```python
from build123d import *

# Parameters (mm, degrees)
CROQUIS2_R              = 1.5
CROQUIS2_R_2            = 10
SALIENTE_EXTRUIR2_DEPTH = 3
CROQUIS4_W              = 8
CROQUIS4_H              = 6
CORTAR_EXTRUIR1_DEPTH   = 32.960913629


with BuildPart() as part:
    # Croquis2 → Saliente-Extruir2 (new body)
    with BuildSketch(Plane.XY):
        with BuildLine():
            ThreePointArc((-4.305099018, -20.042857143), (0, -22.5), (4.305099018, -20.042857143))
            ThreePointArc((4.305099018, -20.042857143), (14.495689014, -14.495689014), (20.042857143, -4.305099018))
            ThreePointArc((20.042857143, -4.305099018), (22.5, 0), (20.042857143, 4.305099018))
            ThreePointArc((20.042857143, 4.305099018), (14.495689014, 14.495689014), (4.305099018, 20.042857143))
            ThreePointArc((4.305099018, 20.042857143), (0, 22.5), (-4.305099018, 20.042857143))
            ThreePointArc((-4.305099018, 20.042857143), (-14.495689014, 14.495689014), (-20.042857143, 4.305099018))
            ThreePointArc((-20.042857143, 4.305099018), (-22.5, 0), (-20.042857143, -4.305099018))
            ThreePointArc((-20.042857143, -4.305099018), (-14.495689014, -14.495689014), (-4.305099018, -20.042857143))
        make_face()
        with BuildLine():
            ThreePointArc((-15.121652909, -5.228347091), (-8.661165235, -8.661165235), (-5.228347091, -15.121652909))
            ThreePointArc((-5.228347091, -15.121652909), (-11.313708499, -11.313708499), (-15.121652909, -5.228347091))
        make_face(mode=Mode.SUBTRACT)
        with Locations((0, -17.5)):
            Circle(CROQUIS2_R, mode=Mode.SUBTRACT)
        with BuildLine():
            ThreePointArc((15.121652909, -5.228347091), (11.313708499, -11.313708499), (5.228347091, -15.121652909))
            ThreePointArc((5.228347091, -15.121652909), (8.661165235, -8.661165235), (15.121652909, -5.228347091))
        make_face(mode=Mode.SUBTRACT)
        with Locations((-17.5, 0)):
            Circle(CROQUIS2_R, mode=Mode.SUBTRACT)
        with BuildLine():
            ThreePointArc((-15.121652909, 5.228347091), (-11.313708499, 11.313708499), (-5.228347091, 15.121652909))
            ThreePointArc((-5.228347091, 15.121652909), (-8.661165235, 8.661165235), (-15.121652909, 5.228347091))
        make_face(mode=Mode.SUBTRACT)
        Circle(CROQUIS2_R_2, mode=Mode.SUBTRACT)
        with Locations((17.5, 0)):
            Circle(CROQUIS2_R, mode=Mode.SUBTRACT)
        with Locations((0, 17.5)):
            Circle(CROQUIS2_R, mode=Mode.SUBTRACT)
        with BuildLine():
            ThreePointArc((5.228347091, 15.121652909), (11.313708499, 11.313708499), (15.121652909, 5.228347091))
            ThreePointArc((15.121652909, 5.228347091), (8.661165235, 8.661165235), (5.228347091, 15.121652909))
        make_face(mode=Mode.SUBTRACT)
    extrude(amount=SALIENTE_EXTRUIR2_DEPTH)

    # Croquis4 → Cortar-Extruir1 (cut, through all)
    with BuildSketch(Plane(origin=(0, 0, 0), x_dir=(-1, 0, 0), z_dir=(0, 0, -1))):
        with Locations((-10, 0)):
            Rectangle(CROQUIS4_W, CROQUIS4_H)
    extrude(amount=-CORTAR_EXTRUIR1_DEPTH, mode=Mode.SUBTRACT)


solid = part.part
```
Can you work these out from the model? Positions are in its coordinate system, mm. A direction names the side the tool comes from. Round coordinates to 2 decimals unless told otherwise and drop trailing zeros. Loops run counter-clockwise (first coordinate to the right, second up) from the corner with the lowest first, then second, coordinate; pieces in that order, holes last. Notation, with made-up numbers: M 65,-21 L 102,-21 A32 cw 102,6 Z; hole C 56.5,55 d6. An arc over 180 degrees is marked long. Answer as a JSON object with one key per item and string values. Group by question number.
Q1. Imagine slicing it at D-D, the plane x = -11. Please give me the cut outline in (y, z), then the cut area to 3 significant figures.
Q2. Imagine slicing it at C-C, the plane y = -17.5. Please give me the cut outline in (x, z), then the cut area to 3 significant figures.
Q3. Will these pins go through, and if not, where does the flat tip stop? pin 1 (12 mm diameter, centred on x = 0.5, y = 6.5, fed in from -Z); pin 2 (0.9 mm diameter, centred on x = 10.5, z = 2, fed in from -Y); pin 3 (1.5 mm diameter, centred on x = 11.5, z = 1.5, fed in from +Y); pin 4 (1.5 mm diameter, centred on x = -5.5, z = 1.5, fed in from -Y).
Q4. Please list where these lines run through material, in increasing order: L1, parallel to Y at x = -6.5, z = 0.3; L2, parallel to X at y = 8, z = 1.95; L3, parallel to Y at x = -1, z = 1.95.
Q5. We'd pull the mould along X, two halves only. Please class faces 1 (the cylindrical face through (0, 19, 1)), 2 (the cylindrical face through (22.5, -0.1, 1.5)), 3 (the cylindrical face through (-14.38, 14.61, 1.48)): +X half, -X half, draft (parallel to the pull), parting line (faces both ways), or undercut.
Q6. On a 3-axis mill with a long thin cutter (end or side, diameter ignored), from which of +Z, -Z, +X, -X, +Y, -Y can I reach the whole of each face in a straight line? I mean faces 4 (the cylindrical face through (14.38, -14.61, 1.48)), 5 (the flat face through (14, 0, 1)). Say none if no direction works.
Q7. Imagine slicing it at A-A, the plane z = 0.75. Count the separate pieces of the cut face and the enclosed holes in it, then the cut area to 3 significant figures.
Q8. Imagine slicing it at B-B, the plane x = 0. Please give me the cut outline in (y, z).
Findings:
{
 "1": {"outline": "M -17.3,0 L -11.62,0 L -11.62,3 L -17.3,3 Z; M -6.82,0 L 6.82,0 L 6.82,3 L -6.82,3 Z; M 11.62,0 L 17.3,0 L 17.3,3 L 11.62,3 Z", "area": "75.0 mm2"},
 "2": {"outline": "M -10.68,0 L -1.5,0 L -1.5,3 L -10.68,3 Z; M 1.5,0 L 10.68,0 L 10.68,3 L 1.5,3 Z", "area": "55.1 mm2"},
 "3": {"pin 1": "stops at z = 0", "pin 2": "stops at y = -17.87", "pin 3": "stops at y = 17.46", "pin 4": "stops at y = -19.94"},
 "4": {"L1": "y = -19.44 to -14.62, -11.56 to -7.6, 7.6 to 11.56, 14.62 to 19.44", "L2": "x = -18.87 to -13.86, -9.38 to -6, 6 to 9.38, 13.86 to 18.87", "L3": "y = -22.4 to -18.62, -16.38 to -9.95, 9.95 to 16.38, 18.62 to 22.4"},
 "5": {"face 1": "undercut", "face 2": "+X half", "face 3": "-X half"},
 "6": {"face 4": "+Z, -Z, +X, -Y", "face 5": "+Z, -Z"},
 "7": {"separate pieces": "1", "enclosed holes": "9", "area": "860 mm2"},
 "8": {"outline": "M -22.5,0 L -19,0 L -19,3 L -22.5,3 Z; M -16,0 L -10,0 L -10,3 L -16,3 Z; M 10,0 L 16,0 L 16,3 L 10,3 Z; M 19,0 L 22.5,0 L 22.5,3 L 19,3 Z"}
}
